from build123d import *

# Parameters (mm, degrees)
EXTRUDE_1_DEPTH           = 10
HOLE_WIZARD_8_0_8_1_D     = 8
HOLE_WIZARD_8_0_8_1_DEPTH = 6.25
HOLE_WIZARD_M41_D         = 4.5
HOLE_WIZARD_M41_DEPTH     = 11
HOLE_WIZARD_M41_TIP       = 1.351936393
HOLE_WIZARD_M42_D         = 4.5
HOLE_WIZARD_M42_DEPTH     = 6.25
M4X0_72_D                 = 3.3
FILLET_2_R                = 10
FILLET_3_R                = 2


with BuildPart() as part:
    # Эскиз1 → Бобышка-Вытянуть1 (new body)
    with BuildSketch(Plane(origin=(0, 0, 0), x_dir=(1, 0, 0), z_dir=(0, 1, 0))):
        with BuildLine():
            Line((67.040100503, -7), (7.959899497, -7))
            ThreePointArc((7.959899497, -7), (-9.658157174, -4.368065934), (0, 10.6))
            Line((0, 10.6), (75, 10.6))
            ThreePointArc((75, 10.6), (84.658157174, -4.368065934), (67.040100503, -7))
        make_face()
        with BuildLine():
            Line((7.562902882, -0.75), (67.437097118, -0.75))
            ThreePointArc((67.437097118, -0.75), (82.6, 0), (67.437097118, 0.75))
            Line((67.437097118, 0.75), (7.562902882, 0.75))
            ThreePointArc((7.562902882, 0.75), (-7.6, 0), (7.562902882, -0.75))
        make_face(mode=Mode.SUBTRACT)
    extrude(amount=EXTRUDE_1_DEPTH)

    # Диаметр отверстия Ø8.0 (8)1
    with Locations(Plane.XY.offset(7)):
        with Locations((27.5, 5), (47.5, 5)):
            Hole(HOLE_WIZARD_8_0_8_1_D / 2, depth=HOLE_WIZARD_8_0_8_1_DEPTH)

    # Отверстие с зазором M41
    with Locations(Plane.XY.offset(-0.75)):
        with Locations((47.5, 5), (27.5, 5)):
            Hole(HOLE_WIZARD_M41_D / 2, depth=HOLE_WIZARD_M41_DEPTH)
            with Locations((0, 0, -(HOLE_WIZARD_M41_DEPTH + HOLE_WIZARD_M41_TIP / 2))):  # 118° drill point
                Cone(0, HOLE_WIZARD_M41_D / 2, HOLE_WIZARD_M41_TIP, mode=Mode.SUBTRACT)

    # Отверстие с зазором M42
    with Locations(Plane.XY.offset(7)):
        with Locations((37.5, 5)):
            Hole(HOLE_WIZARD_M42_D / 2, depth=HOLE_WIZARD_M42_DEPTH)

    # Отверстие обработанное метчиком M4x0.72 (through all)
    with Locations(Plane.XY.offset(-0.75)):
        with Locations((37.5, 5)):
            Hole(M4X0_72_D / 2)

    # Скругление2
    fillet_2_edges = [part.edges().sort_by_distance(p)[0] for p in [
        (67.040100503, 5, 7),
        (7.959899497, 5, 7),
    ]]
    fillet(fillet_2_edges, radius=FILLET_2_R)

    # Скругление3
    fillet_3_edges = [part.edges().sort_by_distance(p)[0] for p in [
        (7.562902882, 5, -0.75),
        (7.562902882, 5, 0.75),
        (67.437097118, 5, 0.75),
        (67.437097118, 5, -0.75),
    ]]
    fillet(fillet_3_edges, radius=FILLET_3_R)


solid = part.part
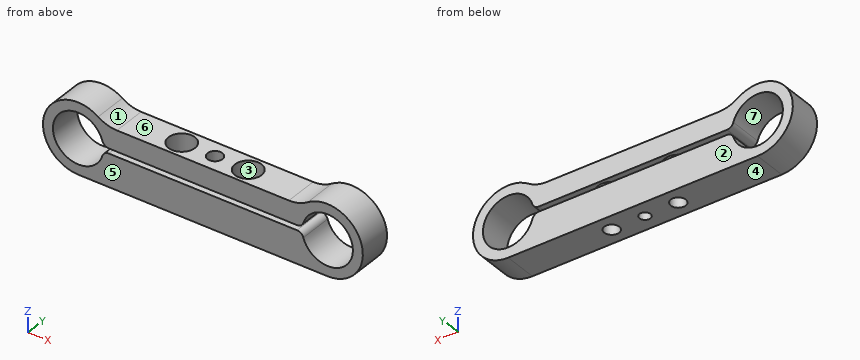
Check sheet for the modelled part. Datum: model origin and axes. Units: mm. Face numbers are marked on the shaded views. A direction names the side the tool comes from. Coordinates: 2 decimals unless noted, no trailing zeros. Loops run counter-clockwise (first coordinate to the right, second up) from the corner with the lowest first, then second, coordinate; pieces in that order, holes last. Notation, with made-up numbers: (33.5, 35) -> (68.5, 35) arc R24 ccw to (68.5, 45) -> close; hole circle Ø11 at (50.25, 11). An arc over 180 degrees is marked (long way). Answer in a Markdown table with one row per item.
1. Sectioned sample at A-A, the plane x = 37.5. Record the boundary of the cut face in (y, z), then the cut area to 3 significant figures.
Check values:
| item | result |
|---|---|
| outline | (0, -10.6) -> (3.35, -10.6) -> (3.35, -0.75) -> (0, -0.75) -> close; (0, 0.75) -> (2.75, 0.75) -> (2.75, 7) -> (0, 7) -> close; (6.65, -10.6) -> (10, -10.6) -> (10, -0.75) -> (6.65, -0.75) -> close; (7.25, 0.75) -> (10, 0.75) -> (10, 7) -> (7.25, 7) -> close |
| area | 100 mm2 |
2. Sectioned sample at C-C, the plane x = 27.5. Record the boundary of the cut face in (y, z).
Check values:
| item | result |
|---|---|
| outline | (0, -10.6) -> (2.75, -10.6) -> (2.75, -0.75) -> (0, -0.75) -> close; (0, 0.75) -> (1, 0.75) -> (1, 7) -> (0, 7) -> close; (7.25, -10.6) -> (10, -10.6) -> (10, -0.75) -> (7.25, -0.75) -> close; (9, 0.75) -> (10, 0.75) -> (10, 7) -> (9, 7) -> close |
3. Sectioned sample at D-D, the plane y = 5. Give the number of separate pieces and of enclosed holes in the cut face, then the cut area to 3 significant figures.
Check values:
| item | result |
|---|---|
| separate pieces | 6 |
| enclosed holes | 0 |
| area | 1,010 mm2 |
4. Material ranges on line 1 along Z through (x, y) = (14, 7.75); line 2 along X through (y, z) = (9, -0.5); line 3 along X through (y, z) = (2, -6), recorded low to high. Write a range as [from, to].
Check values:
| item | result |
|---|---|
| line 1 | z = [-10.6, -0.75], [0.75, 7] |
| line 2 | x = [-10.59, -7.58], [82.58, 85.59] |
| line 3 | x = [-8.74, -4.66], [4.66, 70.34], [79.66, 83.74] |
5. Sectioned sample at B-B, the plane z = -5.5. Record the boundary of the cut face in (x, y) (3 decimals).
Check values:
| item | result |
|---|---|
| outline | (-9.061, 0) -> (-5.245, 0) -> (-5.245, 10) -> (-9.061, 10) -> close; (5.245, 0) -> (69.755, 0) -> (69.755, 10) -> (5.245, 10) -> close; (80.245, 0) -> (84.061, 0) -> (84.061, 10) -> (80.245, 10) -> close; hole circle Ø4.5 at (27.5, 5); hole circle Ø3.3 at (37.5, 5); hole circle Ø4.5 at (47.5, 5) |
6. Go/stop test with flat-tipped pins: pin 1 (4 mm diameter, centred on x = 27.5, y = 5, fed in from +Z); pin 2 (6 mm diameter, centred on x = 47.5, y = 5, fed in from -Z); pin 3 (2 mm diameter, centred on x = 64.5, y = 5, fed in from +Z); pin 4 (3 mm diameter, centred on x = 33, y = 3.5, fed in from +Z). Record where each tip stops, or that it passes through.
Check values:
| item | result |
|---|---|
| pin 1 | passes through |
| pin 2 | stops at z = -10.6 |
| pin 3 | stops at z = 7.23 |
| pin 4 | stops at z = 7 |
7. Release check for a two-part mould opening along Z. For the marked faces 4, 5, 6 and 7 record: released by +Z, released by -Z, zero draft, split by the parting line, or undercut.
Check values:
| item | result |
|---|---|
| face 4 | released by -Z |
| face 5 | zero draft |
| face 6 | released by +Z |
| face 7 | undercut |
8. Access from +Z, -Z, +X, -X, +Y, -Y to the whole of each face (thin tool, end or side, straight path). Record for the marked faces 1, 2 and 3.
Check values:
| item | result |
|---|---|
| face 1 | +Z, +Y, -Y |
| face 2 | +Z, -Z, +X, -X, +Y |
| face 3 | +Z |
